Geometry check sheet. Reference: drawing and pictorial views, mm from the part's lowest x, y, z. A direction names the side the tool comes from. Round coordinates to 2 decimals unless told otherwise and drop trailing zeros. Loops run counter-clockwise (first coordinate to the right, second up) from the corner with the lowest first, then second, coordinate; pieces in that order, holes last. Notation, with made-up numbers: (-4.75, -36) - (1.25, -36) arc R26 ccw to (1.25, -5) - close; hole circle Ø10 at (-23.5, 71.25). An arc over 180 degrees is marked (long way). Put each result on its own line as item: value. Start each with the question number.
Item 1: Section check B-B, the plane x = 2.8. Record the cut outline in (y, z).
Item 2: Material ranges on line 1 along Y through (x, z) = (0.9, 1.3); line 2 along X through (y, z) = (3.25, 2.85); line 3 along Y through (x, z) = (2.5, 3.2), recorded low to high.
Item 3: Draft check along Z on the marked faces 4, 5, 6 and 7. Enter one of: pulls with the +Z half, pulls with the -Z half, needs draft (parallel to the pull), parting line crosses it, or undercut.
Item 4: Tool access check on the marked faces 1, 2 and 3. Record the directions out of +Z, -Z, +X, -X, +Y, -Y that give a thin tool (end or side, any length) a straight path to the whole face; none if there is none.
Item 5: Section check C-C, the plane y = 4.75. Record the cut outline in (x, z).
Item 6: Section check D-D, the plane x = 1.7. Record the cut outline in (y, z).
Item 7: Gauge pin test, flat end, axial feed: pin 1 Ø1.5 at (x, y) = (1, 1) entering from +Z. Record the tip position at first contact, or that the pin passes through.
Item 8: Section check A-A, the plane z = 2.9. Record the cut outline in (x, y), and give its area (3 significant figures).
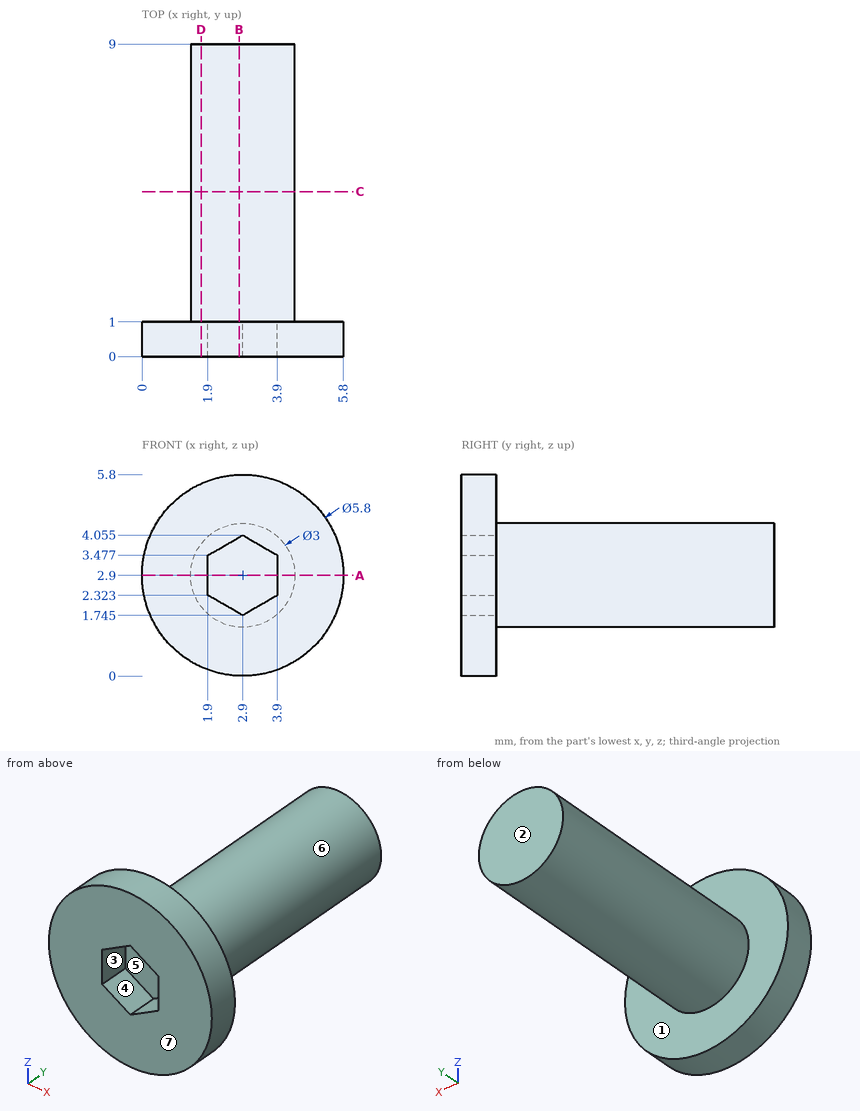
Check result:
1. outline: (0, 0) - (1, 0) - (1, 1.4) - (9, 1.4) - (9, 4.4) - (1, 4.4) - (1, 5.8) - (0, 5.8) - (0, 4) - (1, 4) - (1, 1.8) - (0, 1.8) - close
2. line 1: 0 to 1
2. line 2: 1.4 to 4.4
2. line 3: 1 to 9
3. face 4: undercut
3. face 5: undercut
3. face 6: parting line crosses it
3. face 7: needs draft
4. face 1: +Y
4. face 2: +Z, -Z, +X, -X, +Y
4. face 3: -Y
5. outline: circle Ø3 at (2.9, 2.9)
6. outline: (0, 0.26) - (1, 0.26) - (1, 2) - (9, 2) - (9, 3.8) - (1, 3.8) - (1, 5.54) - (0, 5.54) - close
7. pin 1: z = 5.56
8. outline: (0, 0) - (1.9, 0) - (1.9, 1) - (3.9, 1) - (3.9, 0) - (5.8, 0) - (5.8, 1) - (4.4, 1) - (4.4, 9) - (1.4, 9) - (1.4, 1) - (0, 1) - close
8. area: 27.8 mm²
